Autodesk Inventor part; units mm, degrees
ref_plane "YZ Plane" through (0, 0, 0) normal (1, 0, 0) x (0, 1, 0)
ref_plane "XZ Plane" through (0, 0, 0) normal (0, 1, 0) x (-1, 0, 0)
ref_plane "XY Plane" through (0, 0, 0) normal (0, 0, 1) x (1, 0, 0)
sketch "Sketch1" plane through (0, 0, 0) normal (0, 0, 1) x (1, 0, 0)
  line L0 (-254, -330.2) -> (254, -330.2)
  line L1 (254, -330.2) -> (254, 330.2)
  line L2 (254, 330.2) -> (-254, 330.2)
  line L3 (-254, 330.2) -> (-254, -330.2)
  point P0 (0, 0)
  dimension "d0" = 508
  dimension "d1" = 660.4
  dimension "d2" = 330.2
  dimension "d3" = 254
extrude "Extrusion1" add sketch "Sketch1" along normal blind 1.5875
sketch "Sketch2" plane through (0, 0, 1.5875) normal (0, 0, 1) x (1, 0, 0)
  line L0 (-254, -330.2) -> (-254, 330.2)
  line L1 (254, -330.2) -> (-254, -330.2)
  line L2 (-254, 330.2) -> (254, 330.2)
  circle A0 centre (-82.55, 171.45) radius 146.05
  circle A1 centre (146.05, 50.8) radius 95.25
  arc A2 (-228.6, 50.8) -> (146.05, -323.85) centre (146.05, 50.8) ccw
  line L3 (-228.6, 50.8) -> (-228.6, 203.2)
  line L4 (146.05, -323.85) -> (222.25, -323.85)
  circle A3 centre (146.05, 50.8) radius 14.2875
  circle A4 centre (76.4372, 288.4526) radius 3.175
  circle A5 centre (171.4841, 288.4526) radius 3.175
  line L5 (254, 330.2) -> (254, -330.2)
  point P0 (0, 0)
  point P1 (-82.55, 317.5)
  point P2 (-10.4279, 298.45)
  dimension "d6" = 292.1
  dimension "d7" = 158.75
  dimension "d8" = 171.45
  dimension "d11" = 190.5
  dimension "d16" = 152.4
  dimension "d19" = 76.2
  dimension "d23" = 28.575
  dimension "d27" = 279.4
  dimension "d28" = 25.4
  dimension "d29" = 6.35
  dimension "d31" = 381
  dimension "d33" = 6.35
  dimension "d34" = 6.35
  dimension "d215" = 107.95
extrude "Extrusion2" cut sketch "Sketch2" against normal blind 93.6625 contours A0 | A3
sketch "Sketch10" plane through (0, 0, 1.5875) normal (0, 0, 1) x (1, 0, 0)
  circle A0 centre (146.05, 50.8) radius 14.2875
  line L0 (254, 330.2) -> (254, -330.2)
  circle A1 centre (241.3, 127) radius 3.175
  circle A2 centre (241.3, -25.4) radius 3.175
  circle A3 centre (92.6171, 160.4537) radius 3.175
  line L1 (241.3, -25.4) -> (241.3, 127) construction
  line L2 (241.3, 127) -> (92.6171, 160.4537) construction
  line L3 (146.05, 50.8) -> (241.3, -25.4) construction
  line L4 (146.05, 50.8) -> (241.3, 127) construction
  line L5 (146.05, 50.8) -> (92.6171, 160.4537) construction
  point P0 (0, 0)
  dimension "d208" = 6.35
  dimension "d210" = 12.7
  dimension "d214" = 152.4
extrude "Extrusion10" cut sketch "Sketch10" against normal up to next contours A1 | A2 | A3
sketch "Sketch11" plane through (0, 0, 1.5875) normal (0, 0, 1) x (1, 0, 0)
  line L0 (-254, -330.2) -> (-254, 330.2)
  line L1 (254, -330.2) -> (-254, -330.2)
  line L2 (-254, -330.2) -> (-254, -171.45) construction
  line L3 (-254, -171.45) -> (-95.25, -330.2) construction
  line L4 (-254, -330.2) -> (-95.25, -330.2) construction
  circle A0 centre (-209.0987, -162.4697) radius 3.175
  circle A1 centre (-130.1559, -241.4125) radius 3.175
  circle A2 centre (-51.2132, -320.3553) radius 3.175
  line L5 (-209.0987, -162.4697) -> (-130.1559, -241.4125) construction
  line L6 (-130.1559, -241.4125) -> (-51.2132, -320.3553) construction
  line L7 (-254, -171.45) -> (-217.3278, -134.7778) construction
  point P0 (0, 0)
  dimension "d216" = 158.75
  dimension "d217" = 158.75
  dimension "d218" = 6.35
  dimension "d219" = 38.1
  dimension "d220" = 25.4
extrude "Extrusion11" cut sketch "Sketch11" against normal up to next
properties part number "Shooter Plate"
Geometry check sheet. Reference: the model listing, model coordinates, mm. Coordinates: 2 decimals unless noted, no trailing zeros. Loops run counter-clockwise (first coordinate to the right, second up) from the corner with the lowest first, then second, coordinate; pieces in that order, holes last.
Item 1: Sectioned sample at B-B, the plane y = 171.45. Record the boundary of the cut face in (x, z), then the cut area to 3 significant figures.
Item 2: Release check for a two-part mould opening along Y. For faces 1 (the face through (-101.563, 316.257, 0.805)), 2 (the face through (131.776, 51.428, 0.805)), 3 (the face through (-4, -69, 1.588)) record: released by +Y, released by -Y, zero draft, split by the parting line, or undercut.
Item 3: Thickness scan on line 1 (Y direction, x = 241.3, z = 0.3) (3 decimals); line 2 (Y direction, x = 146.05, z = 0.75); line 3 (X direction, y = 171.45, z = 1.15). Record the ranges inside material, lowest first.
Item 4: Sectioned sample at C-C, the plane y = 50.8. Record the boundary of the cut face in (x, z), then the cut area to 3 significant figures.
Item 5: Sectioned sample at A-A, the plane x = 146.05. Record the boundary of the cut face in (y, z).
Item 6: Sectioned sample at D-D, the plane z = 0.5. Count the separate pieces of the cut face and the enclosed holes in it, then the cut area to 3 significant figures.
Check result:
1. outline: (-254, 0) - (-228.6, 0) - (-228.6, 1.59) - (-254, 1.59) - close; (63.5, 0) - (254, 0) - (254, 1.59) - (63.5, 1.59) - close
1. area: 343 mm2
2. face 1: undercut
2. face 2: undercut
2. face 3: zero draft
3. line 1: y = -330.2 to -28.575, -22.225 to 123.825, 130.175 to 330.2
3. line 2: y = -330.2 to 36.51, 65.09 to 330.2
3. line 3: x = -254 to -228.6, 63.5 to 254
4. outline: (-254, 0) - (-164.86, 0) - (-164.86, 1.59) - (-254, 1.59) - close; (-0.24, 0) - (131.76, 0) - (131.76, 1.59) - (-0.24, 1.59) - close; (160.34, 0) - (254, 0) - (254, 1.59) - (160.34, 1.59) - close
4. area: 500 mm2
5. outline: (-330.2, 0) - (36.51, 0) - (36.51, 1.59) - (-330.2, 1.59) - close; (65.09, 0) - (330.2, 0) - (330.2, 1.59) - (65.09, 1.59) - close
6. separate pieces: 1
6. enclosed holes: 8
6. area: 268,000 mm2
